Could you check a few things on this drawing? It's one solid part, dimensions in mm from its lowest x, y, z. A direction names the side the tool comes from. Coordinates: 2 decimals unless noted, no trailing zeros. Loops run counter-clockwise (first coordinate to the right, second up) from the corner with the lowest first, then second, coordinate; pieces in that order, holes last.
1) Imagine slicing it at B-B on x = 55. Please give me the cut outline in (y, z).
2) If I drill on line 1 along X through (y, z) = (56, 35.5); line 2 along Z through (x, y) = (3.5, 15); line 3 along Y through (x, z) = (34.5, 19), over which ranges is the centre line in solid material (lowest first)?
3) Imagine slicing it at D-D on z = 25. Please give me the cut outline in (x, y).
4) For the marked faces 4, 5, 6 and 7, which set-ups out of +Z, -Z, +X, -X, +Y, -Y let a thin tool reach every point of the face, with its end or its side?
5) Imagine slicing it at A-A on y = 15. Please give me the cut outline in (x, z).
6) Thinking about a two-plate mould opening in X: for the marked faces 1, 2 and 3, which applies, released by +X, released by -X, zero draft, split by the parting line, or undercut?
7) Imagine slicing it at C-C on z = 30.5. Please give me the cut outline in (x, y).
8) Will these pins go through, and if not, where does the flat tip stop? P1, Ø1.5, axis at x = 20, z = 18.5, coming from the -Y side; P2, Ø7.5, axis at y = 53, z = 10, coming from the +X side; P3, Ø6, axis at x = 66.5, y = 40.5, coming from the -Z side; P4, Ø16, axis at x = 35, y = 30, coming from the +Z side.
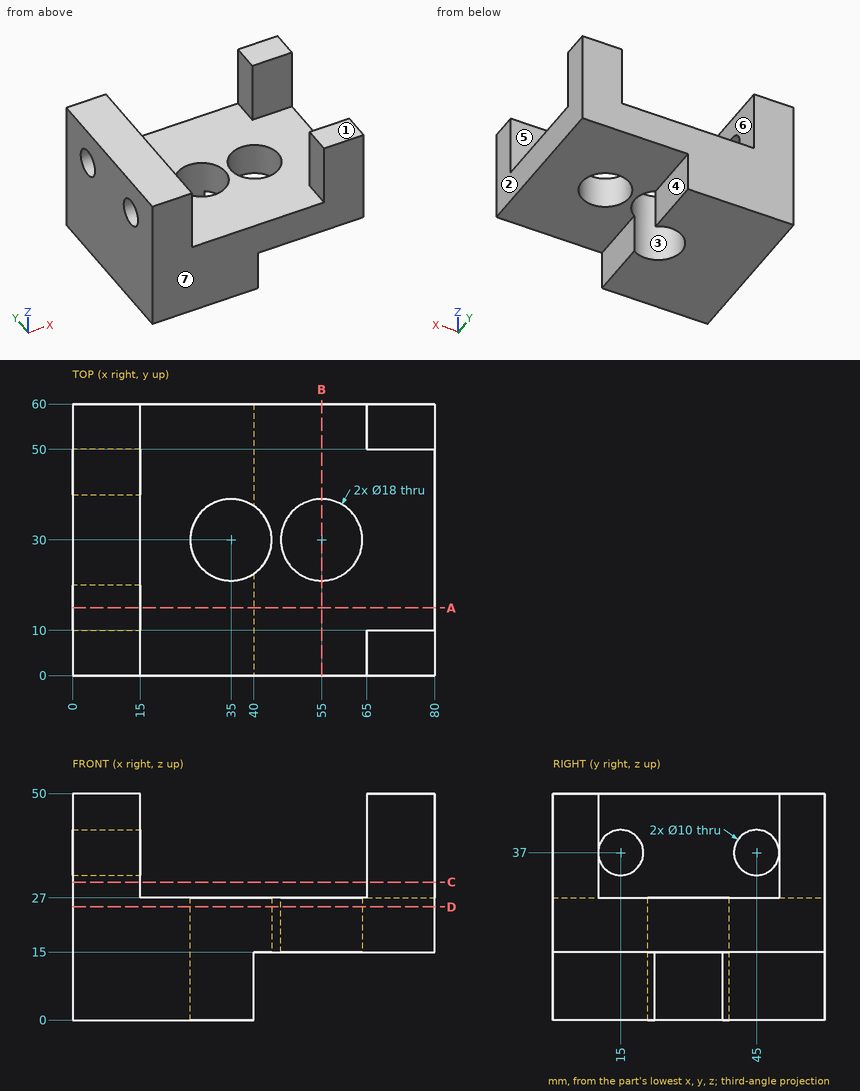
Filled in:
1. outline: (0, 15) - (21, 15) - (21, 27) - (0, 27) - close; (39, 15) - (60, 15) - (60, 27) - (39, 27) - close
2. line 1: x = 0 to 15, 65 to 80
2. line 2: z = 0 to 32, 42 to 50
2. line 3: y = 0 to 21.01, 38.99 to 60
3. outline: (0, 0) - (80, 0) - (80, 60) - (0, 60) - close; hole circle Ø18 at (35, 30); hole circle Ø18 at (55, 30)
4. face 4: -Z, +X, +Y, -Y
4. face 5: +Z, +X
4. face 6: +Z, +Y, -Y
4. face 7: +Z, -Z, +X, -X, -Y
5. outline: (0, 0) - (40, 0) - (40, 15) - (80, 15) - (80, 27) - (15, 27) - (15, 32) - (0, 32) - close; (0, 42) - (15, 42) - (15, 50) - (0, 50) - close
6. face 1: zero draft
6. face 2: released by +X
6. face 3: undercut
7. outline: (0, 0) - (15, 0) - (15, 60) - (0, 60) - close; (65, 0) - (80, 0) - (80, 10) - (65, 10) - close; (65, 50) - (80, 50) - (80, 60) - (65, 60) - close
8. P1: stops at y = 0
8. P2: stops at x = 40
8. P3: stops at z = 15
8. P4: passes through
